Geometry: see drawing. Coordinates: mm, zero at the bounding-box minimum. A direction names the side the tool comes from. Give positions to 0.01 mm unless a question says otherwise; leave off trailing zeros. Write each loop counter-clockwise with the first axis right and the second up, starting at its lowest first coordinate (ties: lowest second). Pieces come first, ordered by that corner, then holes. Notation, with made-up numbers: (57.25, -1) -> (92.25, -1) arc R11 ccw to (92.25, 8) -> close; hole circle Ø8 at (63, -25.5). An arc over 180 degrees is marked (long way). Use CSV: the item, a comma, the result in double quotes. Start each with the question number.
1) Draft query along X for the marked faces 1, 2 and 3. Return one class per face: pulls with the +X half, pulls with the -X half, needs draft (parallel to the pull), parting line crosses it, or undercut.
2) Set-up query: the marked faces 4 and 5. Return all of +Z, -Z, +X, -X, +Y, -Y with unobstructed straight access to the full face (end or side cutting, diameter ignored); none if empty.
3) Section D-D (x = 1.45). Output: boundary loops of the cut face in (y, z).
4) Material intervals for line 1 (Y direction, x = 1.4, z = 5.25); line 2 (X direction, y = 2.7, z = 4.5); line 3 (Y direction, x = 2.4, z = 6.5), sorted ascending. Write a range as [from, to].
5) Section B-B (y = 3.25). Output: boundary loops of the cut face in (x, z), plus the area to 3 significant figures.
6) Section A-A (z = 7.5). Count the separate pieces of the cut face and the enclosed holes in it.
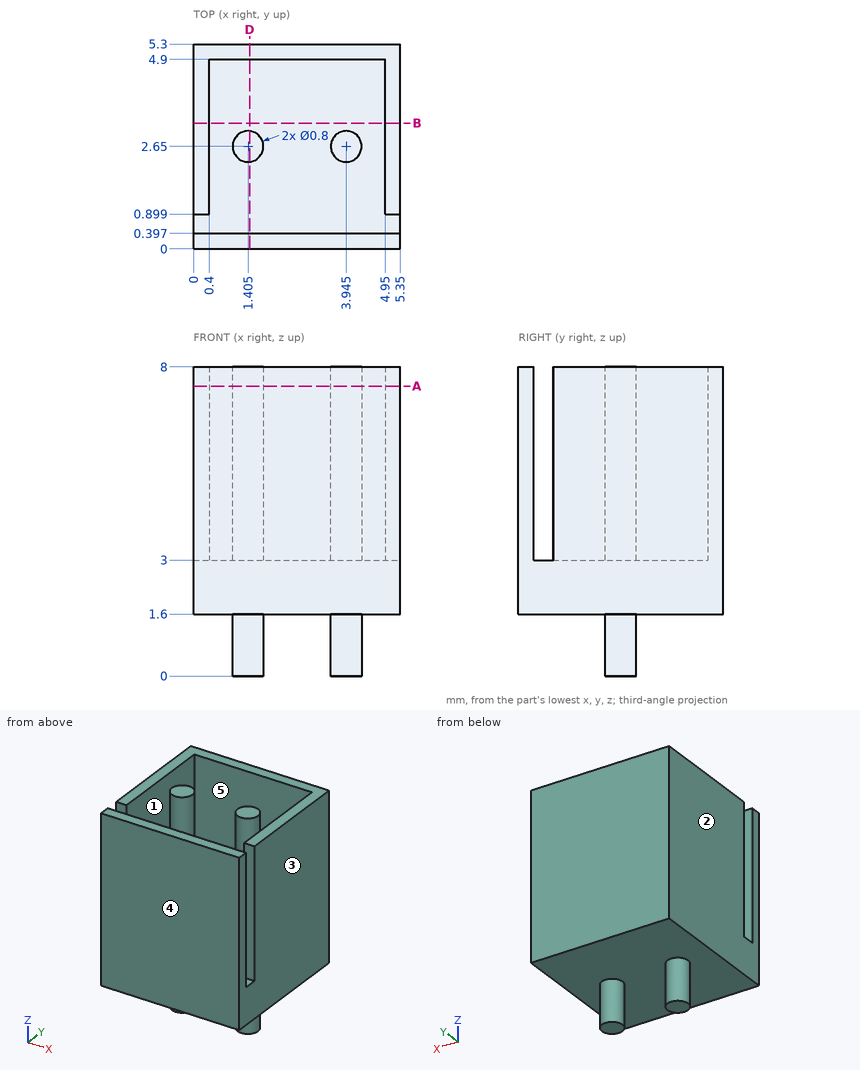
Answers follow:
1,face 1,"undercut"
1,face 2,"pulls with the -X half"
1,face 3,"pulls with the +X half"
2,face 4,"+Z, -Z, +X, -X, -Y"
2,face 5,"+Z"
3,outline,"(0, 1.6) -> (2.25, 1.6) -> (2.25, 0) -> (3.05, 0) -> (3.05, 1.6) -> (5.3, 1.6) -> (5.3, 8) -> (4.9, 8) -> (4.9, 3) -> (3.05, 3) -> (3.05, 8) -> (2.25, 8) -> (2.25, 3) -> (0.4, 3) -> (0.4, 8) -> (0, 8) -> close"
4,line 1,"y = [0, 0.4], [2.25, 3.05], [4.9, 5.3]"
4,line 2,"x = [0, 0.4], [1.01, 1.8], [3.55, 4.34], [4.95, 5.35]"
4,line 3,"y = [0, 0.4], [4.9, 5.3]"
5,outline,"(0, 1.6) -> (5.35, 1.6) -> (5.35, 8) -> (4.95, 8) -> (4.95, 3) -> (0.4, 3) -> (0.4, 8) -> (0, 8) -> close"
5,area,"11.5 mm^2"
6,separate pieces,"4"
6,enclosed holes,"0"
